from build123d import *

# Parameters (mm, degrees)
SKETCH1_R           = 2.77876
SKETCH1_R_2         = 7.62
SKETCH1_R_3         = 3.81
BOSS_EXTRUDE1_DEPTH = 6.35


with BuildPart() as part:
    # Sketch1 → Boss-Extrude1 (new body)
    with BuildSketch(Plane(origin=(0, 0, 0), x_dir=(1, 0, 0), z_dir=(0, 1, 0))):
        with BuildLine():
            Line((-15.875, -26.6065), (15.875, -26.6065))
            Line((15.875, -26.6065), (15.875, -16.237330354))
            ThreePointArc((15.875, -16.237330354), (15.176911953, -13.667262721), (13.274508805, -11.803546858))
            Line((13.274508805, -11.803546858), (9.161857046, -9.503624849))
            ThreePointArc((9.161857046, -9.503624849), (7.9255795, -7.853183269), (8.321289158, -5.829386481))
            ThreePointArc((8.321289158, -5.829386481), (10.156557189, 0.264473195), (8.006627428, 6.254559715))
            ThreePointArc((8.006627428, 6.254559715), (7.477616777, 8.035735763), (8.302840532, 9.700501853))
            Line((8.302840532, 9.700501853), (14.205887505, 15.048906872))
            ThreePointArc((14.205887505, 15.048906872), (15.439012733, 16.75449557), (15.875, 18.81351129))
            Line((15.875, 18.81351129), (15.875, 26.6065))
            Line((15.875, 26.6065), (-15.875, 26.6065))
            Line((-15.875, 26.6065), (-15.875, 18.81351129))
            ThreePointArc((-15.875, 18.81351129), (-15.439012733, 16.75449557), (-14.205887505, 15.048906872))
            Line((-14.205887505, 15.048906872), (-8.302840532, 9.700501853))
            ThreePointArc((-8.302840532, 9.700501853), (-7.477616777, 8.035735763), (-8.006627428, 6.254559715))
            ThreePointArc((-8.006627428, 6.254559715), (-10.156557189, 0.264473195), (-8.321289158, -5.829386481))
            ThreePointArc((-8.321289158, -5.829386481), (-7.9255795, -7.853183269), (-9.161857046, -9.503624849))
            Line((-9.161857046, -9.503624849), (-13.274508805, -11.803546858))
            ThreePointArc((-13.274508805, -11.803546858), (-15.176911953, -13.667262721), (-15.875, -16.237330354))
            Line((-15.875, -16.237330354), (-15.875, -26.6065))
        make_face()
        with Locations(Location((11.0109, 21.5265, 0), (0, 0, 270))):
            Circle(SKETCH1_R, mode=Mode.SUBTRACT)
        with Locations(Location((11.0109, -18.9865, 0), (0, 0, 270))):
            Circle(SKETCH1_R, mode=Mode.SUBTRACT)
        with Locations(Location((-11.0109, -18.9865, 0), (0, 0, 90))):
            Circle(SKETCH1_R, mode=Mode.SUBTRACT)
        with Locations(Location((-11.0109, 21.5265, 0), (0, 0, 90))):
            Circle(SKETCH1_R, mode=Mode.SUBTRACT)
        with Locations(Location((0, 0, 0), (0, 0, 270))):
            Circle(SKETCH1_R_2, mode=Mode.SUBTRACT)
        with Locations(Location((0, 15.875, 0), (0, 0, 270))):
            Circle(SKETCH1_R_3, mode=Mode.SUBTRACT)
        with Locations(Location((0, -15.875, 0), (0, 0, 270))):
            Circle(SKETCH1_R_3, mode=Mode.SUBTRACT)
    extrude(amount=BOSS_EXTRUDE1_DEPTH)


solid = part.part
Can you work these out from the model? Positions are in its coordinate system, mm. A direction names the side the tool comes from. Coordinates: 2 decimals unless noted, no trailing zeros. Order: outer loops, then holes, each group sorted by start corner. A loop starts at its lowest first (then second) coordinate and runs counter-clockwise, first axis right, second up. Notation, with made-up numbers: (58, -29.5) -> (90, -29.5) arc R32 ccw to (90, 2.5) -> close; hole circle Ø3 at (43.25, 51). An arc over 180 degrees is marked (long way). Use one line per item in the form item = value.
Q1. Imagine slicing it at A-A, the plane z = 0. List the corners of the cut face in (x, y) for me.
From the geometry:
outline = (-10.16, 0) -> (-7.62, 0) -> (-7.62, 6.35) -> (-10.16, 6.35) -> close; (7.62, 0) -> (10.16, 0) -> (10.16, 6.35) -> (7.62, 6.35) -> close
Q2. Imagine slicing it at D-D, the plane y = 1.5. List the corners of the cut face in (x, z) for me (1 decimal).
From the geometry:
outline = (-15.9, -26.6) -> (15.9, -26.6) -> (15.9, -18.8) arc R5.1 ccw to (14.2, -15) -> (8.3, -9.7) arc R2.5 cw to (8, -6.3) arc R10.2 ccw to (8.3, 5.8) arc R2.5 cw to (9.2, 9.5) -> (13.3, 11.8) arc R5.1 ccw to (15.9, 16.2) -> (15.9, 26.6) -> (-15.9, 26.6) -> (-15.9, 16.2) arc R5.1 ccw to (-13.3, 11.8) -> (-9.2, 9.5) arc R2.5 cw to (-8.3, 5.8) arc R10.2 ccw to (-8, -6.3) arc R2.5 cw to (-8.3, -9.7) -> (-14.2, -15) arc R5.1 ccw to (-15.9, -18.8) -> close; hole circle Ø5.6 at (-11, -21.5); hole circle Ø5.6 at (-11, 19); hole circle Ø15.2 at (0, 0); hole circle Ø7.6 at (0, -15.9); hole circle Ø7.6 at (0, 15.9); hole circle Ø5.6 at (11, -21.5); hole circle Ø5.6 at (11, 19)
Q3. Imagine slicing it at B-B, the plane x = 0. Give the number of separate pieces and of enclosed holes in the cut face, then the cut area to 3 significant figures.
From the geometry:
separate_pieces = 4
enclosed_holes = 0
area = 144 mm²
Q4. We'd pull the mould along X, two halves only. Please class faces 4 (the face through (7.555, 3.131, -0.992)), 5 (the face through (-11.296, 3.131, -12.412)), 6 (the face through (15.875, 3, -23)): released by +X, released by -X, zero draft, split by the parting line, or undercut.
From the geometry:
face_4 = undercut
face_5 = released by -X
face_6 = released by +X
Q5. I need wall thicknesses on L1, parallel to X at y = 2.75, z = 0; L2, parallel to X at y = 2.25, z = -20 (3 decimals); L3, parallel to Z at x = 1, y = 2.5. Which ranges of each line are inside material? Lowest first, please.
From the geometry:
L1 = -10.16 to -7.62, 7.62 to 10.16
L2 = -15.875 to -13.333, -8.689 to 8.689, 13.333 to 15.875
L3 = -26.61 to -19.55, -12.2 to -7.55, 7.55 to 12.2, 19.55 to 26.61
Q6. Which directions (+Z, -Z, +X, -X, +Y, -Y) give clear straight access to the entire face, cutting with the end or side of a thin tool? Please do faces 1 (the face through (13.354, 3.131, 20.48)), 2 (the face through (-15.45, 3.13, -16.78)), 3 (the face through (15.196, 3.131, 13.7)).
From the geometry:
face_1 = +Y, -Y
face_2 = -X, +Y, -Y
face_3 = +X, +Y, -Y
Q7. Imagine slicing it at C-C, the plane x = -5.5. List the corners of the cut face in (y, z) for me.
From the geometry:
outline = (0, -26.61) -> (6.35, -26.61) -> (6.35, -5.27) -> (0, -5.27) -> close; (0, 5.27) -> (6.35, 5.27) -> (6.35, 26.61) -> (0, 26.61) -> close
Q8. Will these pins go through, and if not, where does the flat tip stop? P1, Ø5, axis at x = 11.01, z = -21.53, coming from the +Y side; P2, Ø1.5, axis at y = 3, z = -7.5, coming from the -X side.
From the geometry:
P1 = through
P2 = -7.7
